Autodesk Inventor part; units mm, degrees
ref_plane "YZ Plane" through (0, 0, 0) normal (1, 0, 0) x (0, 1, 0)
ref_plane "XZ Plane" through (0, 0, 0) normal (0, 1, 0) x (-1, 0, 0)
ref_plane "XY Plane" through (0, 0, 0) normal (0, 0, 1) x (1, 0, 0)
sketch "Sketch1" plane through (0, 0, 0) normal (1, 0, 0) x (0, 1, 0)
  arc A0 (12.7, -5.2436) -> (12.7, -6.3485) centre (12.7, -5.796) ccw
  line L0 (12.7, -5.2436) -> (12.7, -4.1904)
  arc A1 (12.7, -4.1904) -> (11.7608, -3.2512) centre (11.7608, -4.1904) ccw
  line L1 (11.7608, -3.2512) -> (11.4294, -3.2512)
  arc A2 (11.4294, -3.2512) -> (10.4902, -4.1904) centre (11.4294, -4.1904) ccw
  line L2 (10.4902, -4.1904) -> (10.4902, -6.3485)
  arc A3 (8.6665, -7.1039) -> (10.4902, -6.3485) centre (9.4219, -6.3485) ccw
  line L3 (8.6665, -7.1039) -> (5.2999, -3.7373)
  arc A4 (4.6482, -2.164) -> (5.2999, -3.7373) centre (6.8732, -2.164) ccw
  line L4 (4.6482, -2.164) -> (4.6482, 2.164)
  arc A5 (5.2999, 3.7373) -> (4.6482, 2.164) centre (6.8732, 2.164) ccw
  line L5 (8.6665, 7.1039) -> (5.2999, 3.7373)
  arc A6 (10.4902, 6.3485) -> (8.6665, 7.1039) centre (9.4219, 6.3485) ccw
  line L6 (10.4902, 4.1904) -> (10.4902, 6.3485)
  arc A7 (10.4902, 4.1904) -> (11.4294, 3.2512) centre (11.4294, 4.1904) ccw
  line L7 (11.7608, 3.2512) -> (11.4294, 3.2512)
  arc A8 (11.7608, 3.2512) -> (12.7, 4.1904) centre (11.7608, 4.1904) ccw
  line L8 (12.7, 5.2436) -> (12.7, 4.1904)
  arc A9 (12.7, 6.3485) -> (12.7, 5.2436) centre (12.7, 5.796) ccw
  line L9 (12.7, 9.8037) -> (12.7, 6.3485)
  arc A10 (12.58, 10.8954) -> (12.7, 9.8037) centre (12.7, 10.3562) ccw
  arc A11 (12.58, 10.8954) -> (10.8954, 12.58) centre (10.1173, 10.1173) ccw
  arc A12 (9.8037, 12.7) -> (10.8954, 12.58) centre (10.3562, 12.7) ccw
  line L10 (6.3485, 12.7) -> (9.8037, 12.7)
  arc A13 (5.2436, 12.7) -> (6.3485, 12.7) centre (5.796, 12.7) ccw
  line L11 (4.1904, 12.7) -> (5.2436, 12.7)
  arc A14 (4.1904, 12.7) -> (3.2512, 11.7608) centre (4.1904, 11.7608) ccw
  line L12 (3.2512, 11.4294) -> (3.2512, 11.7608)
  arc A15 (3.2512, 11.4294) -> (4.1904, 10.4902) centre (4.1904, 11.4294) ccw
  line L13 (6.3485, 10.4902) -> (4.1904, 10.4902)
  arc A16 (7.1039, 8.6665) -> (6.3485, 10.4902) centre (6.3485, 9.4219) ccw
  line L14 (3.7373, 5.2999) -> (7.1039, 8.6665)
  arc A17 (2.164, 4.6482) -> (3.7373, 5.2999) centre (2.164, 6.8732) ccw
  line L15 (-2.164, 4.6482) -> (2.164, 4.6482)
  arc A18 (-3.7373, 5.2999) -> (-2.164, 4.6482) centre (-2.164, 6.8732) ccw
  line L16 (-3.7373, 5.2999) -> (-7.1039, 8.6665)
  arc A19 (-6.3485, 10.4902) -> (-7.1039, 8.6665) centre (-6.3485, 9.4219) ccw
  line L17 (-6.3485, 10.4902) -> (-4.1904, 10.4902)
  arc A20 (-4.1904, 10.4902) -> (-3.2512, 11.4294) centre (-4.1904, 11.4294) ccw
  line L18 (-3.2512, 11.4294) -> (-3.2512, 11.7608)
  arc A21 (-3.2512, 11.7608) -> (-4.1904, 12.7) centre (-4.1904, 11.7608) ccw
  line L19 (-4.1904, 12.7) -> (-5.2436, 12.7)
  arc A22 (-6.3485, 12.7) -> (-5.2436, 12.7) centre (-5.796, 12.7) ccw
  line L20 (-6.3485, 12.7) -> (-9.8037, 12.7)
  arc A23 (-10.8954, 12.58) -> (-9.8037, 12.7) centre (-10.3562, 12.7) ccw
  arc A24 (-10.8954, 12.58) -> (-12.58, 10.8954) centre (-10.1173, 10.1173) ccw
  arc A25 (-12.7, 9.8037) -> (-12.58, 10.8954) centre (-12.7, 10.3562) ccw
  line L21 (-12.7, 9.8037) -> (-12.7, 6.3485)
  arc A26 (-12.7, 5.2436) -> (-12.7, 6.3485) centre (-12.7, 5.796) ccw
  line L22 (-12.7, 5.2436) -> (-12.7, 4.1904)
  arc A27 (-12.7, 4.1904) -> (-11.7608, 3.2512) centre (-11.7608, 4.1904) ccw
  line L23 (-11.7608, 3.2512) -> (-11.4294, 3.2512)
  arc A28 (-11.4294, 3.2512) -> (-10.4902, 4.1904) centre (-11.4294, 4.1904) ccw
  line L24 (-10.4902, 4.1904) -> (-10.4902, 6.3485)
  arc A29 (-8.6665, 7.1039) -> (-10.4902, 6.3485) centre (-9.4219, 6.3485) ccw
  line L25 (-8.6665, 7.1039) -> (-5.2999, 3.7373)
  arc A30 (-4.6482, 2.164) -> (-5.2999, 3.7373) centre (-6.8732, 2.164) ccw
  line L26 (-4.6482, -2.164) -> (-4.6482, 2.164)
  arc A31 (-5.2999, -3.7373) -> (-4.6482, -2.164) centre (-6.8732, -2.164) ccw
  line L27 (-8.6665, -7.1039) -> (-5.2999, -3.7373)
  arc A32 (-10.4902, -6.3485) -> (-8.6665, -7.1039) centre (-9.4219, -6.3485) ccw
  line L28 (-10.4902, -4.1904) -> (-10.4902, -6.3485)
  arc A33 (-10.4902, -4.1904) -> (-11.4294, -3.2512) centre (-11.4294, -4.1904) ccw
  line L29 (-11.7608, -3.2512) -> (-11.4294, -3.2512)
  arc A34 (-11.7608, -3.2512) -> (-12.7, -4.1904) centre (-11.7608, -4.1904) ccw
  line L30 (-12.7, -5.2436) -> (-12.7, -4.1904)
  arc A35 (-12.7, -6.3485) -> (-12.7, -5.2436) centre (-12.7, -5.796) ccw
  line L31 (-12.7, -9.8037) -> (-12.7, -6.3485)
  arc A36 (-12.58, -10.8954) -> (-12.7, -9.8037) centre (-12.7, -10.3562) ccw
  arc A37 (-12.58, -10.8954) -> (-10.8954, -12.58) centre (-10.1173, -10.1173) ccw
  arc A38 (-9.8037, -12.7) -> (-10.8954, -12.58) centre (-10.3562, -12.7) ccw
  line L32 (-6.3485, -12.7) -> (-9.8037, -12.7)
  arc A39 (-5.2436, -12.7) -> (-6.3485, -12.7) centre (-5.796, -12.7) ccw
  line L33 (-4.1904, -12.7) -> (-5.2436, -12.7)
  arc A40 (-4.1904, -12.7) -> (-3.2512, -11.7608) centre (-4.1904, -11.7608) ccw
  line L34 (-3.2512, -11.4294) -> (-3.2512, -11.7608)
  arc A41 (-3.2512, -11.4294) -> (-4.1904, -10.4902) centre (-4.1904, -11.4294) ccw
  line L35 (-6.3485, -10.4902) -> (-4.1904, -10.4902)
  arc A42 (-7.1039, -8.6665) -> (-6.3485, -10.4902) centre (-6.3485, -9.4219) ccw
  line L36 (-3.7373, -5.2999) -> (-7.1039, -8.6665)
  arc A43 (-2.164, -4.6482) -> (-3.7373, -5.2999) centre (-2.164, -6.8732) ccw
  line L37 (-2.164, -4.6482) -> (2.164, -4.6482)
  arc A44 (3.7373, -5.2999) -> (2.164, -4.6482) centre (2.164, -6.8732) ccw
  line L38 (3.7373, -5.2999) -> (7.1039, -8.6665)
  arc A45 (6.3485, -10.4902) -> (7.1039, -8.6665) centre (6.3485, -9.4219) ccw
  line L39 (6.3485, -10.4902) -> (4.1904, -10.4902)
  arc A46 (4.1904, -10.4902) -> (3.2512, -11.4294) centre (4.1904, -11.4294) ccw
  line L40 (3.2512, -11.4294) -> (3.2512, -11.7608)
  arc A47 (3.2512, -11.7608) -> (4.1904, -12.7) centre (4.1904, -11.7608) ccw
  line L41 (4.1904, -12.7) -> (5.2436, -12.7)
  arc A48 (6.3485, -12.7) -> (5.2436, -12.7) centre (5.796, -12.7) ccw
  line L42 (6.3485, -12.7) -> (9.8037, -12.7)
  arc A49 (10.8954, -12.58) -> (9.8037, -12.7) centre (10.3562, -12.7) ccw
  arc A50 (10.8954, -12.58) -> (12.58, -10.8954) centre (10.1173, -10.1173) ccw
  arc A51 (12.7, -9.8037) -> (12.58, -10.8954) centre (12.7, -10.3562) ccw
  line L43 (12.7, -9.8037) -> (12.7, -6.3485)
  circle A52 centre (0, 0) radius 2.6035
  point P0 (0, 0)
  point P1 (0, 0)
extrude "Extrusion1" add sketch "Sketch1" against normal blind 255
properties part number "horizontalStrut" material "Aluminum 6061"
The model under review builds one solid part; all positions refer to its coordinate system, in mm. A direction names the side the tool comes from. Give positions to 0.01 mm unless a question says otherwise; leave off trailing zeros. Write each loop counter-clockwise with the first axis right and the second up, starting at its lowest first coordinate (ties: lowest second). Pieces come first, ordered by that corner, then holes. Notation, with made-up numbers: M -11,-13 L 37,-13 A19 ccw 37,4 Z; hole C 43.5,24.5 d6. An arc over 180 degrees is marked long. One line per question, with ' | ' between items. Start each with the question number.
Item 1: For faces 1 (the flat face through (-126, 0, 4.648)), 2 (the flat face through (-126, 4.648, 0)), 3 (the flat face through (0, -3, 0)), list the 3-axis set-ups (+Z, -Z, +X, -X, +Y, -Y) from which the entire face can be reached by the end or side of a thin tool; tool diameter is ignored.
Item 2: Draft analysis for pull direction Z (two halves, no side actions). For faces 4 (the flat face through (-126, 0, -4.648)), 5 (the flat face through (-255, -3, 0)), 6 (the flat face through (-126, -4.648, 0)), state which applies: released by +Z, released by -Z, zero draft, split by the parting line, or undercut.
Item 3: Wall thickness on line 1 (Z direction, x = -55, y = 0); line 2 (Y direction, x = -53.5, z = -9.5); line 3 (Y direction, x = -178, z = 6.75): over which ranges is each line inside the solid? List them lowest first. Write a range as from..to.
Item 4: We need section A-A on y = 0. Write out the cut boundary in (x, z).
Item 5: For pin 1 (1.7 mm diameter, centred on x = -175.5, y = -5.5, fed in from -Z); pin 2 (3.5 mm diameter, centred on x = -178.5, z = -1, fed in from -Y); pin 3 (4 mm diameter, centred on x = -194, z = -2, fed in from -Y); pin 4 (3.5 mm diameter, centred on x = -127.5, y = -1, fed in from -Z), all flat-tipped, find the tip position at first contact; note any pin that passes through.
Results found:
1) face 1: +Z, +X, -X | face 2: +X, -X, +Y | face 3: +Z, -Z, +X, +Y, -Y
2) face 4: released by -Z | face 5: zero draft | face 6: undercut
3) line 1: z = -4.65..-2.6, 2.6..4.65 | line 2: y = -12.7..-7.41, 7.41..12.7 | line 3: y = -12.7..-10.41, -8.31..-5.19, 5.19..8.31, 10.41..12.7
4) outline: M -255,-4.65 L 0,-4.65 L 0,-2.6 L -255,-2.6 Z; M -255,2.6 L 0,2.6 L 0,4.65 L -255,4.65 Z
5) pin 1: stops at z = -12.7 | pin 2: stops at y = -4.73 | pin 3: stops at y = -12.68 | pin 4: stops at z = -4.73
